Input: part model. Units: mm. Frame: model coordinates. Face numbers are marked on the shaded views. A direction names the side the tool comes from. Round coordinates to 2 decimals unless told otherwise and drop trailing zeros. Order: outer loops, then holes, each group sorted by start corner. A loop starts at its lowest first (then second) coordinate and runs counter-clockwise, first axis right, second up. Notation, with made-up numbers: (-17.5, -34.75) -> (23.5, -34.75) arc R31 cw to (23.5, -10.75) -> close; hole circle Ø5 at (-23.75, -3). An arc over 180 degrees is marked (long way). Answer as CSV lines item,"result". Start each with the question number.
1) Mould query, pull axis X, two halves, no side actions, for the marked faces 4, 5 and 6. Classes: +X half, -X half, draft (parallel to the pull), parting line (faces both ways), or undercut.
2) Section query B-B, the plane z = 7.5. Output: boundary loops of the cut face in (x, y).
3) Line query: L1, parallel to X at y = 49, z = 8.75; L2, parallel to Y at x = -6, z = 3; L3, parallel to Z at x = 17.75, y = 0.7. Output: solid intervals per line, ascending.
4) First-contact query: P1, Ø2, axis at y = 19.5, z = 8, coming from the +X side; P2, Ø8, axis at y = 36.5, z = 8.5, coming from the -X side; P3, Ø4, axis at x = 20.5, z = 9, coming from the +Y side; P4, Ø2.5, axis at x = -17.75, z = 7.5, coming from the -Y side. Flat tips, straight axial feed; report the tip coordinate or a pass-through.
5) Section query D-D, the plane z = 10.75. Output: boundary loops of the cut face in (x, y).
6) Access query for the marked faces 1, 2 and 3. Directions: +Z, -Z, +X, -X, +Y, -Y. A direction counts if a zero-diameter tool reaches every point of the face in a straight line with its end or side. Return the directions, or none.
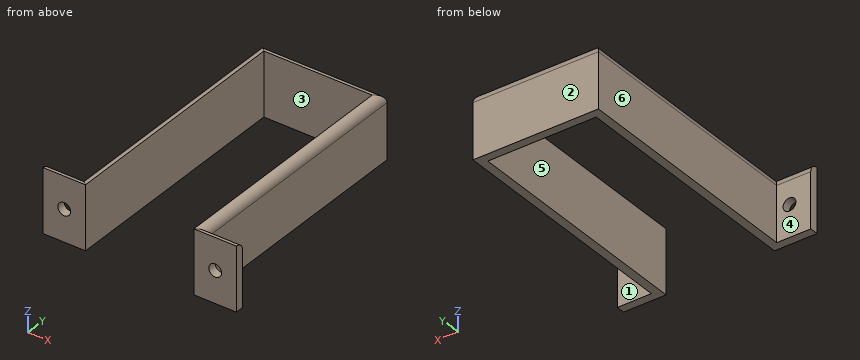
```python
from build123d import *

# Parameters (mm, degrees)
F1_DEPTH = 15
F2_R     = 1.5
F3_DEPTH = 2
F4_R     = 1.99999


# Not quite as in the source:
# - a fillet or chamfer is up to 0.001 mm smaller than in the source, because OpenCascade refuses the exact size


with BuildPart() as f1:
    # F0 (on Top) → F1 (new body)
    with BuildSketch(Plane.XY):
        Polygon((-22.75, 2), (-22.75, 0), (-12.75, 0), (-12.75, 57), (0, 57), (12.75, 57), (12.75, 0), (22.75, 0), (22.75, 2), (14.75, 2), (14.75, 59), (0, 59), (-14.75, 59), (-14.75, 2), align=None)
    extrude(amount=F1_DEPTH)

    # F2 (on Front) → F3 (cut)
    with BuildSketch(Plane.XZ):
        with Locations((-17.75, 7.5)):
            Circle(F2_R)
        with Locations((17.75, 7.5)):
            Circle(F2_R)
    extrude(amount=-F3_DEPTH, mode=Mode.SUBTRACT)

    # F4 (radius 2 in the source; OpenCascade refuses exactly that, so slightly less here)
    f4_edges = [f1.edges().sort_by_distance(p)[0] for p in [
        (-14.75, 30.5, 15),
        (0, 59, 15),
        (14.75, 30.5, 15),
        (18.75, 2, 15),
        (-18.75, 2, 15),
    ]]
    fillet(f4_edges, radius=F4_R)


solid = f1.part
```
Findings:
1,face 4,"draft"
1,face 5,"undercut"
1,face 6,"-X half"
2,outline,"(-22.75, 0) -> (-19.25, 0) -> (-19.25, 2) -> (-22.75, 2) -> close; (-16.25, 0) -> (-12.75, 0) -> (-12.75, 57) -> (12.75, 57) -> (12.75, 0) -> (16.25, 0) -> (16.25, 2) -> (14.75, 2) -> (14.75, 59) -> (-14.75, 59) -> (-14.75, 2) -> (-16.25, 2) -> close; (19.25, 0) -> (22.75, 0) -> (22.75, 2) -> (19.25, 2) -> close"
3,L1,"x = -14.75 to -12.75, 12.75 to 14.75"
3,L2,"y = 57 to 59"
3,L3,"z = 0 to 6, 9 to 14.87"
4,P1,"stops at x = 14.75"
4,P2,"stops at x = -14.75"
4,P3,"stops at y = 2"
4,P4,"passes through"
5,outline,"(-22.75, 0) -> (-12.75, 0) -> (-12.75, 57) -> (12.75, 57) -> (12.75, 0) -> (22.75, 0) -> (22.75, 2) -> (14.75, 2) -> (14.75, 59) -> (-14.75, 59) -> (-14.75, 2) -> (-22.75, 2) -> close"
6,face 1,"+Z, -Z, +X, +Y"
6,face 2,"+Z, -Z, +X, -X, +Y"
6,face 3,"+Z, -Z, -Y"
